```python
from build123d import *

# Parameters (mm, degrees)
F0_W     = 20.7835333422
F0_H     = 16.9197171926
F0_W_2   = 23.7798653543
F0_H_2   = 18.441430293
F1_DEPTH = 211.2
F2_DEPTH = 167.2


with BuildPart() as f1:
    # F0 (on Front) → F1 (new body)
    with BuildSketch(Plane.XZ):
        with Locations((-19.4875816815, 14.9991363287)):
            Rectangle(F0_W, F0_H)
        Polygon((-9.0958150104, 6.5392777324), (-29.8793483526, 6.5392777324), (-29.8793483526, -11.9021525607), (17.4585692585, -11.9021525607), (17.4585692585, 6.5392777324), align=None)
        Polygon((17.4585692585, -11.9021525607), (-29.8793483526, -11.9021525607), (-29.8793483526, -25.1875463873), (41.2384346128, -25.1875463873), (41.2384346128, -11.9021525607), align=None)
        Polygon((41.2384346128, 23.458994925), (-9.0958150104, 23.458994925), (-9.0958150104, 6.5392777324), (17.4585692585, 6.5392777324), (41.2384346128, 6.5392777324), align=None)
        with Locations((29.3485019356, -2.6814374141)):
            Rectangle(F0_W_2, F0_H_2)
    extrude(amount=-F1_DEPTH)

    # F0 (on Front) → F2 (cut)
    with BuildSketch(Plane.XZ):
        Polygon((41.2384346128, 23.458994925), (-9.0958150104, 23.458994925), (-9.0958150104, 6.5392777324), (17.4585692585, 6.5392777324), (41.2384346128, 6.5392777324), align=None)
        with Locations((29.3485019356, -2.6814374141)):
            Rectangle(F0_W_2, F0_H_2)
    extrude(amount=-F2_DEPTH, mode=Mode.SUBTRACT)


solid = f1.part
```
Model file for the job. Use its own axes, mm. A direction names the side the tool comes from. Coordinates: 2 decimals unless noted, no trailing zeros. Write each loop counter-clockwise with the first axis right and the second up, starting at its lowest first coordinate (ties: lowest second). Pieces come first, ordered by that corner, then holes. Notation, with made-up numbers: (-6, 63) - (38, 63) arc R15 ccw to (38, 74) - close; hole circle Ø6 at (48, 83.25). An arc over 180 degrees is marked (long way). One line per item, written item: value. Start each with the question number.
1. Slice it at B-B (x = 36.5). Write the cut outline in (y, z).
2. Slice it at C-C (z = -7). Write the cut outline in (x, y).
3. Flat gauge pins, fed straight in: pin 1 (12 mm diameter, centred on x = 24.5, y = 46.5, fed in from +Z); pin 2 (13.5 mm diameter, centred on y = 84, z = 18, fed in from +X); pin 3 (2 mm diameter, centred on x = -2.5, y = 128, fed in from +Z). Where does each tip first touch, or does it go through?
4. Slice it at A-A (y = 85.5). Write the cut outline in (x, z).
5. Tool access for faces 1 (the flat face through (4, 82, 6.539)), 2 (the flat face through (-10, 128, 23.459)): list every direction of +Z, -Z, +X, -X, +Y, -Y with a clear straight run to the whole face (end or side of a thin tool).
6. Probe line 1 (X direction, y = 53, z = 18); line 2 (Y direction, x = 11, z = 10); line 3 (X direction, y = 130, z = -10). List the from-to ranges inside material, lowest first. Write a range as from..to.
Answers below:
1. outline: (0, -25.19) - (211.2, -25.19) - (211.2, 23.46) - (167.2, 23.46) - (167.2, -11.9) - (0, -11.9) - close
2. outline: (-29.88, 0) - (17.46, 0) - (17.46, 167.2) - (41.24, 167.2) - (41.24, 211.2) - (-29.88, 211.2) - close
3. pin 1: stops at z = -11.9
3. pin 2: stops at x = -9.1
3. pin 3: stops at z = 6.54
4. outline: (-29.88, -25.19) - (41.24, -25.19) - (41.24, -11.9) - (17.46, -11.9) - (17.46, 6.54) - (-9.1, 6.54) - (-9.1, 23.46) - (-29.88, 23.46) - close
5. face 1: +Z, +X, -Y
5. face 2: +Z, +X, -X, +Y, -Y
6. line 1: x = -29.88..-9.1
6. line 2: y = 167.2..211.2
6. line 3: x = -29.88..17.46
